```python
from build123d import *

# Parameters (mm, degrees)
SKETCH_1_W      = 20
SKETCH_1_H      = 20
EXTRUDE_1_DEPTH = 70
SKETCH_2_W      = 20
SKETCH_2_H      = 20
EXTRUDE_2_DEPTH = 10
SKETCH_4_R      = 30
SKETCH_4_R_2    = 25
EXTRUDE_5_DEPTH = 10
SKETCH_6_R      = 25
EXTRUDE_6_DEPTH = 10


with BuildPart() as part:
    # Sketch 1 → Extrude 1 (new body)
    with BuildSketch(Plane(origin=(0, 0, 0), x_dir=(1, 0, 0), z_dir=(0, 1, 0))):
        Rectangle(SKETCH_1_W, SKETCH_1_H)
    extrude(amount=-EXTRUDE_1_DEPTH)

    # Sketch 2 → Extrude 2 (add)
    with BuildSketch(Plane(origin=(10, 0, 0), x_dir=(0, 0, -1), z_dir=(1, 0, 0))):
        with Locations((0, -70)):
            Rectangle(SKETCH_2_W, SKETCH_2_H)
    extrude(amount=EXTRUDE_2_DEPTH)



with BuildPart() as body_2:
    # Sketch 4 → Extrude 5 (new body)
    with BuildSketch(Plane(origin=(20, 0, 0), x_dir=(0, 0, -1), z_dir=(1, 0, 0))):
        with Locations((0, -70)):
            Circle(SKETCH_4_R)
        with Locations((0, -70)):
            Circle(SKETCH_4_R_2, mode=Mode.SUBTRACT)
    extrude(amount=EXTRUDE_5_DEPTH)


with BuildPart() as part_1:
    add(part.part)

    add(body_2.part)  # Extrude 6 merges body 2
    # Sketch 6 → Extrude 6 (add)
    with BuildSketch(Plane(origin=(20, 0, 0), x_dir=(0, 0, -1), z_dir=(1, 0, 0))):
        with Locations((0, -70)):
            Circle(SKETCH_6_R)
    extrude(amount=EXTRUDE_6_DEPTH)


solid = part_1.part
```
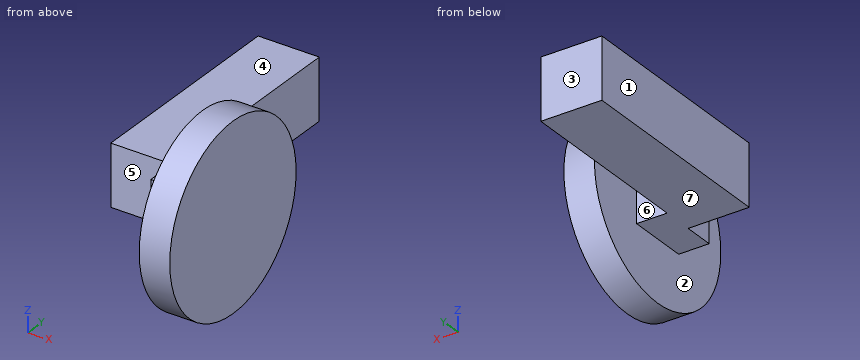
For this review, take the finished solid that the model builds, in its own axes (mm). Face numbers are marked on the shaded views. A direction names the side the tool comes from. Coordinates: 2 decimals unless noted, no trailing zeros. Order: outer loops, then holes, each group sorted by start corner. A loop starts at its lowest first (then second) coordinate and runs counter-clockwise, first axis right, second up. Notation, with made-up numbers: (63, 49) -> (75, 49) arc R11 ccw to (75, 66) -> close; hole circle Ø3 at (20, 76). An arc over 180 degrees is marked (long way). Use CSV: the item, a comma, the result in double quotes. Start each with the question number.
Item 1: Wall thickness on probe 1 along Y at (x, z) = (8, 6); probe 2 along Y at (x, z) = (14, -1); probe 3 along X at (y, z) = (-46.5, 0): over which ranges is each line inside the solid? List them lowest first.
Item 2: We need section A-A, the plane y = -59. Give the boundary of the cut face in (x, z), then the cut area to 3 significant figures.
Item 3: We need section D-D, the plane y = -44. Give the boundary of the cut face in (x, z).
Item 4: For the marked faces 4, 5, 6 and 7, list the 3-axis set-ups (+Z, -Z, +X, -X, +Y, -Y) from which the entire face can be reached by the end or side of a thin tool; tool diameter is ignored.
Item 5: We need section C-C, the plane x = 13.5. Give the boundary of the cut face in (y, z), then the cut area to 3 significant figures.
Item 6: Insertion check: pin 1 (5 mm diameter, centred on x = 13.5, z = 0.5, fed in from +Y); pin 2 (5 mm diameter, centred on x = 13, z = 4, fed in from -Y); pin 3 (8 mm diameter, centred on x = 16.5, y = -50.5, fed in from -Z); pin 4 (1 mm diameter, centred on x = 11.5, y = -33, fed in from +Z). Each pin has a flat end and moves straight along its axis. Give the tip position at first contact, or say it passes through.
Item 7: We need section B-B, the plane z = 0. Give the boundary of the cut face in (x, y).
Item 8: Draft analysis for pull direction X (two halves, no side actions). For the marked faces 1, 2 and 3, state which applies: pulls with the +X half, pulls with the -X half, needs draft (parallel to the pull), parting line crosses it, or undercut.
Derived:
1,probe 1,"y = -70 to 0"
1,probe 2,"y = -80 to -60"
1,probe 3,"x = -10 to 10, 20 to 30"
2,outline,"(-10, -10) -> (10, -10) -> (10, 10) -> (-10, 10) -> close; (20, -27.91) -> (30, -27.91) -> (30, 27.91) -> (20, 27.91) -> close"
2,area,"958 mm^2"
3,outline,"(-10, -10) -> (10, -10) -> (10, 10) -> (-10, 10) -> close; (20, -14.97) -> (30, -14.97) -> (30, 14.97) -> (20, 14.97) -> close"
4,face 4,"+Z, -X, +Y, -Y"
4,face 5,"+Z, -Z, -X, -Y"
4,face 6,"+Z, -Z, +Y"
4,face 7,"-Z, -X, +Y, -Y"
5,outline,"(-80, -10) -> (-60, -10) -> (-60, 10) -> (-80, 10) -> close"
5,area,"400 mm^2"
6,pin 1,"stops at y = -60"
6,pin 2,"stops at y = -80"
6,pin 3,"stops at z = -24.32"
6,pin 4,"passes through"
7,outline,"(-10, -70) -> (10, -70) -> (10, -80) -> (20, -80) -> (20, -100) -> (30, -100) -> (30, -40) -> (20, -40) -> (20, -60) -> (10, -60) -> (10, 0) -> (-10, 0) -> close"
8,face 1,"pulls with the -X half"
8,face 2,"undercut"
8,face 3,"needs draft"
